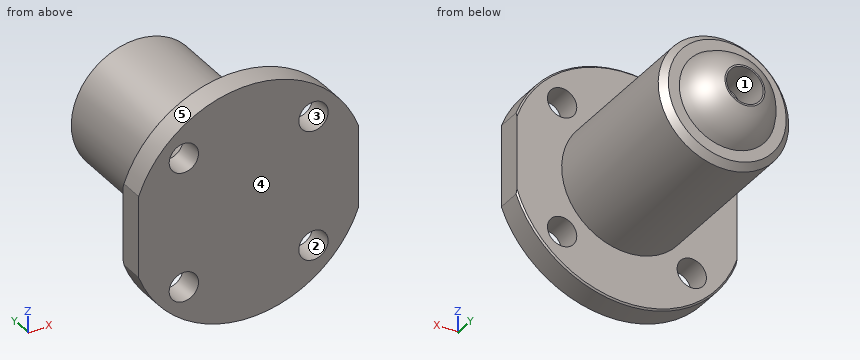
```python
from build123d import *

# Parameters (mm, degrees)
SKETCH_2_R          = 2.5
CUT_EXTRUDE_1_DEPTH = 5
SKETCH_3_R          = 2
CUT_EXTRUDE_2_DEPTH = 5
CHAMFER_1_SIZE      = 0.2


with BuildPart() as part:
    # 草图1 → 旋转1 (revolve)
    with BuildSketch(Plane.XY, mode=Mode.PRIVATE) as revolve_1_sk:
        with BuildLine():
            Line((0, 0), (16, 0))
            Line((16, 0), (16, 3.5))
            Line((16, 3.5), (8.9, 3.5))
            Line((8.9, 3.5), (8.9, 25.138348415))
            Line((8.9, 25.138348415), (8.038348415, 26))
            Line((8.038348415, 26), (6.538348415, 26))
            ThreePointArc((6.538348415, 26), (5.032803689, 28.365273582), (2.719834554, 29.95))
            Line((2.719834554, 29.95), (0, 29.95))
            Line((0, 29.95), (0, 0))
        make_face()
    revolve(revolve_1_sk.sketch.rotate(Axis((0, 33.582842794, 0), (0, -1, 0)), 90), axis=Axis((0, 33.582842794, 0), (0, -1, 0)))

    # 草图2 → 切除-拉伸1 (cut)
    with BuildSketch(Plane(origin=(0, 29.95, 0), x_dir=(1, 0, 0), z_dir=(0, 1, 0))):
        with Locations(Location((0, 0, 0), (0, 0, 270))):
            Circle(SKETCH_2_R)
    extrude(amount=-CUT_EXTRUDE_1_DEPTH, mode=Mode.SUBTRACT)

    # 草图3 → 切除-拉伸2 (cut)
    with BuildSketch(Plane(origin=(0, 3.5, 0), x_dir=(1, 0, 0), z_dir=(0, 1, 0))):
        with Locations(Location((8.838834765, 8.838834765, 0), (0, 0, 270))):
            Circle(SKETCH_3_R)
        with Locations(Location((8.838834765, -8.838834765, 0), (0, 0, 270))):
            Circle(SKETCH_3_R)
        with Locations(Location((-8.838834765, -8.838834765, 0), (0, 0, 270))):
            Circle(SKETCH_3_R)
        with Locations(Location((-8.838834765, 8.838834765, 0), (0, 0, 270))):
            Circle(SKETCH_3_R)
        with BuildLine():
            Line((-15, 5.567764363), (-15, -5.567764363))
            ThreePointArc((-15, -5.567764363), (-16, 0), (-15, 5.567764363))
        make_face()
        with BuildLine():
            Line((15, 5.567764363), (15, -5.567764363))
            ThreePointArc((15, -5.567764363), (16, 0), (15, 5.567764363))
        make_face()
    extrude(amount=-CUT_EXTRUDE_2_DEPTH, mode=Mode.SUBTRACT)

    # 倒角1
    chamfer_1_edges = [part.edges().sort_by_distance(p)[0] for p in [
        (0, 3.5, -16),
        (0, 3.5, 16),
    ]]
    chamfer(chamfer_1_edges, length=CHAMFER_1_SIZE)


solid = part.part
```
Part model, mm, in its own coordinate system. Face numbers are marked on the shaded views. A direction names the side the tool comes from. Round coordinates to 2 decimals unless told otherwise and drop trailing zeros. Loops run counter-clockwise (first coordinate to the right, second up) from the corner with the lowest first, then second, coordinate; pieces in that order, holes last. Notation, with made-up numbers: (-19.5, 34.5) -> (39.5, 34.5) arc R16 ccw to (39.5, 39.5) -> close; hole circle Ø3 at (-23, 66.25). An arc over 180 degrees is marked (long way). Use a Markdown table: item, result.
1) Drop flat-ended pins along their axis: pin 1 Ø1 at (y, z) = (10, -7) entering from -X; pin 2 Ø2.5 at (x, z) = (0.5, 0.5) entering from +Y; pin 3 Ø4.5 at (x, z) = (-8.84, 8.84) entering from +Y. Give the stop position or say it passes through.
The answers:
| item | result |
|---|---|
| pin 1 | stops at x = -6.08 |
| pin 2 | stops at y = 24.95 |
| pin 3 | stops at y = 3.5 |
2) Pull direction Z, two halves, no side cores. Call the marked faces 3, 4 and 5: pulls with the +Z half, pulls with the -Z half, needs draft (parallel to the pull), parting line crosses it, or undercut.
The answers:
| item | result |
|---|---|
| face 3 | undercut |
| face 4 | needs draft |
| face 5 | pulls with the +Z half |
3) Cut at A-A, the plane x = 0. List the corners of the cut face in (y, z).
The answers:
| item | result |
|---|---|
| outline | (0, -16) -> (3.3, -16) -> (3.5, -15.8) -> (3.5, -8.9) -> (25.14, -8.9) -> (26, -8.04) -> (26, -6.54) arc R7 ccw to (29.95, -2.72) -> (29.95, -2.5) -> (24.95, -2.5) -> (24.95, 2.5) -> (29.95, 2.5) -> (29.95, 2.72) arc R7 ccw to (26, 6.54) -> (26, 8.04) -> (25.14, 8.9) -> (3.5, 8.9) -> (3.5, 15.8) -> (3.3, 16) -> (0, 16) -> close |
4) Cut at B-B, the plane y = 2.25. List the corners of the cut face in (x, z), and give its area (3 significant figures).
The answers:
| item | result |
|---|---|
| outline | (-15, -5.57) arc R16 ccw to (15, -5.57) -> (15, 5.57) arc R16 ccw to (-15, 5.57) -> close; hole circle Ø4 at (-8.84, -8.84); hole circle Ø4 at (-8.84, 8.84); hole circle Ø4 at (8.84, -8.84); hole circle Ø4 at (8.84, 8.84) |
| area | 739 mm2 |
5) Tool access for the marked faces 1 and 2: list every direction of +Z, -Z, +X, -X, +Y, -Y with a clear straight run to the whole face (end or side of a thin tool).
The answers:
| item | result |
|---|---|
| face 1 | +Y |
| face 2 | +Y, -Y |
6) Probe line 1 (Y direction, x = -8.5, z = -6); line 2 (Y direction, x = -2, z = 7.5); line 3 (X direction, y = 26.75, z = -1). List the from-to ranges inside material, lowest first. Write a range as [from, to].
The answers:
| item | result |
|---|---|
| line 1 | y = [0, 3.5] |
| line 2 | y = [0, 26] |
| line 3 | x = [-6.12, -2.29], [2.29, 6.12] |
7) Cut at C-C, the plane z = 0. List the corners of the cut face in (x, y).
The answers:
| item | result |
|---|---|
| outline | (-15, 0) -> (15, 0) -> (15, 3.5) -> (8.9, 3.5) -> (8.9, 25.14) -> (8.04, 26) -> (6.54, 26) arc R7 ccw to (2.72, 29.95) -> (2.5, 29.95) -> (2.5, 24.95) -> (-2.5, 24.95) -> (-2.5, 29.95) -> (-2.72, 29.95) arc R7 ccw to (-6.54, 26) -> (-8.04, 26) -> (-8.9, 25.14) -> (-8.9, 3.5) -> (-15, 3.5) -> close |
8) Cut at D-D, the plane z = -10. State how many separate pieces and enclosed holes the cut face has, and give its area (3 significant figures).
The answers:
| item | result |
|---|---|
| separate pieces | 3 |
| enclosed holes | 0 |
| area | 64.6 mm2 |
